Build history of the part. All positions in model axes, mm. A direction names the side the tool comes from. Give positions to 0.01 mm unless a question says otherwise; leave off trailing zeros. Order: outer loops, then holes, each group sorted by start corner. A loop starts at its lowest first (then second) coordinate and runs counter-clockwise, first axis right, second up. Notation, with made-up numbers: M 18,-29.75 L 76,-29.75 A24 ccw 76,0.25 Z; hole C 81,62 d10. An arc over 180 degrees is marked long. Use CSV: the item, a comma, the result in double quotes. Start each with the question number.
Item 1: Band-saw the part on C-C on y = -8. Write the cut outline in (x, z), plus the area to 3 significant figures.
Item 2: Which spindle directions (+Z, -Z, +X, -X, +Y, -Y) get a long thin tool onto all of the face, cutting with end or side? Do faces 1 (the flat face through (0, -216, -10)), 2 (the flat face through (-83, -100, 0)), 3 (the flat face through (75.95, -85, 0)). Say none if no direction does.
Item 3: Two-plate mould, pull along Y, no slides. Class faces 4 (the cylindrical face through (-1.429, -224.984, -0.14)), 5 (the flat face through (86, 96, 0)), 6 (the flat face through (65, -120, -6)): pulls with the +Y half, pulls with the -Y half, needs draft (parallel to the pull), parting line crosses it, or undercut.
Item 4: Pin check, flat tips, straight feed: P1, Ø10, axis at x = 7, z = -27, coming from the +Y side; P2, Ø1.4, axis at y = -86.5, z = -30, coming from the +X side; P3, Ø1, axis at x = 8, y = -124, coming from the -Z side. Stop position of each tip, or through.
Item 5: Band-saw the part on A-A on x = 0. Write the cut outline in (y, z).
Item 6: Band-saw the part on B-B on z = 1. Write the cut outline in (x, y), plus the area to 3 significant figures.
Item 7: Wall check: line 1 along Y through (x, z) = (-76.5, 5); line 2 along Z through (x, y) = (-83, 23.5); line 3 along Z through (x, y) = (52, -156.5). Give the ranges that are in metal, low to high.
Item 8: Band-saw the part on D-D on z = -19.5. Write the cut outline in (x, y).
from build123d import *

# Parameters (mm, degrees)
SKETCH_1_W          = 200
SKETCH_1_H          = 200
EXTRUDE_1_DEPTH     = 10
SKETCH_2_W          = 20.05
SKETCH_2_H          = 20.05
CUT_EXTRUDE_2_DEPTH = 40
SKETCH_5_W          = 130
SKETCH_5_H          = 20
EXTRUDE_2_DEPTH     = 60
EXTRUDE_3_DEPTH     = 20
CUT_EXTRUDE_4_DEPTH = 16
SKETCH_10_W         = 110
SKETCH_10_H         = 10
EXTRUDE_5_DEPTH     = 38
EXTRUDE_6_DEPTH     = 10
EXTRUDE_7_DEPTH     = 120


with BuildPart() as part:
    # 草图1 → 凸台-拉伸1 (new, symmetric)
    with BuildSketch(Plane.XY):
        Rectangle(SKETCH_1_W, SKETCH_1_H)
    extrude(amount=EXTRUDE_1_DEPTH, both=True)

    # 草图2 → 切除-拉伸2 (cut)
    with BuildSketch(Plane(origin=(0, 0, -10), x_dir=(-1, 0, 0), z_dir=(0, 0, -1))):
        with Locations((-85.975, 85.975)):
            Rectangle(SKETCH_2_W, SKETCH_2_H)
        with Locations((85.025, 85.975)):
            Rectangle(SKETCH_2_W, SKETCH_2_H)
        with Locations((85.025, -84.975)):
            Rectangle(SKETCH_2_W, SKETCH_2_H)
        with Locations((-85.975, -84.975)):
            Rectangle(SKETCH_2_W, SKETCH_2_H)
    extrude(amount=-CUT_EXTRUDE_2_DEPTH, mode=Mode.SUBTRACT)

    # 草图5 → 凸台-拉伸2 (add)
    with BuildSketch(Plane.XZ.offset(100)):
        Rectangle(SKETCH_5_W, SKETCH_5_H)
    extrude(amount=EXTRUDE_2_DEPTH)

    # 草图6 → 凸台-拉伸3 (add)
    with BuildSketch(Plane(origin=(0, 0, -10), x_dir=(-1, 0, 0), z_dir=(0, 0, -1))):
        with BuildLine():
            Line((-65, -160), (65, -160))
            ThreePointArc((65, -160), (0, -225), (-65, -160))
        make_face()
    extrude(amount=-EXTRUDE_3_DEPTH)

    # 草图7 → 切除-拉伸4 (cut)
    with BuildSketch(Plane(origin=(0, 0, -10), x_dir=(-1, 0, 0), z_dir=(0, 0, -1))):
        with BuildLine():
            Line((-55, -100), (-55, -80.5))
            Line((-55, -80.5), (55, -80.5))
            Line((55, -80.5), (55, -100))
            Line((55, -100), (55, -160))
            ThreePointArc((55, -160), (0, -215), (-55, -160))
            Line((-55, -160), (-55, -100))
        make_face()
    extrude(amount=-CUT_EXTRUDE_4_DEPTH, mode=Mode.SUBTRACT)

    # 草图10 → 凸台-拉伸5 (add)
    with BuildSketch(Plane(origin=(0, 0, 6), x_dir=(-1, 0, 0), z_dir=(0, 0, -1))):
        with Locations((0, -85.5)):
            Rectangle(SKETCH_10_W, SKETCH_10_H)
    extrude(amount=EXTRUDE_5_DEPTH)

    # 草图11 → 凸台-拉伸6 (add)
    with BuildSketch(Plane(origin=(55, 0, 0), x_dir=(0, 0, -1), z_dir=(1, 0, 0))):
        Polygon((32, -80.5), (10, -80.5), (10, -160), align=None)
    extrude_6 = extrude(amount=EXTRUDE_6_DEPTH)

    # 镜向1: 凸台-拉伸6 across plane
    add(extrude_6.mirror(Plane(origin=(0, 0, 0), x_dir=(0, 0, 1), z_dir=(1, 0, 0))))

    # 草图12 → 凸台-拉伸7 (add)
    with BuildSketch(Plane(origin=(-55, 0, 0), x_dir=(0, 0, -1), z_dir=(1, 0, 0))):
        Polygon((-6, -125.5), (-6, -90.5), (23, -90.5), align=None)
    extrude(amount=EXTRUDE_7_DEPTH)


solid = part.part
Model answer:
1,outline,"M -100,-10 L 100,-10 L 100,10 L -100,10 Z"
1,area,"4,000 mm^2"
2,face 1,"-Z, +X, -X, -Y"
2,face 2,"+Z, -Z, -X, -Y"
2,face 3,"+Z, -Z"
3,face 4,"pulls with the -Y half"
3,face 5,"undercut"
3,face 6,"needs draft"
4,P1,"stops at y = -80.5"
4,P2,"stops at x = 65"
4,P3,"stops at z = 4.34"
5,outline,"M -225,-10 L -215,-10 L -215,6 L -125.5,6 L -90.5,-23 L -90.5,-32 L -80.5,-32 L -80.5,-10 L 100,-10 L 100,10 L -225,10 Z"
6,outline,"M -100,-100 L -65,-100 L -65,-160 A65 ccw 65,-160 L 65,-100 L 100,-100 L 100,100 L -100,100 Z; hole M -95.05,-95 L -75,-95 L -75,-74.95 L -95.05,-74.95 Z; hole M -95.05,75.95 L -75,75.95 L -75,96 L -95.05,96 Z; hole M -55,-160 A55 ccw 55,-160 L 55,-119.47 L -55,-119.47 Z; hole M 75.95,-95 L 96,-95 L 96,-74.95 L 75.95,-74.95 Z; hole M 75.95,75.95 L 96,75.95 L 96,96 L 75.95,96 Z"
6,area,"43,600 mm^2"
7,line 1,"y = -100 to -95, -74.95 to 75.95, 96 to 100"
7,line 2,"z = -10 to 10"
7,line 3,"z = 6 to 10"
8,outline,"M -65,-125.67 L -55,-125.67 L -55,-94.72 L 55,-94.72 L 55,-125.67 L 65,-125.67 L 65,-80.5 L -65,-80.5 Z"
